```python
from build123d import *

# Parameters (mm, degrees)
F1_DEPTH = 6.35
F2_R     = 15.875
F2_R_2   = 8.7674107973
F3_DEPTH = 6.35


# Not quite as in the source:
# - a feature names something its author has since deleted; it is built from what else it names


with BuildPart() as f1:
    # F0 (on Front) → F1 (new body)
    with BuildSketch(Plane.XZ):
        Polygon((-15.875, 25.1552741975), (-50.8, 8.7795666171), (-50.8, -35.6704333829), (0, -35.6704333829), (0, 25.1552741975), align=None)
        Polygon((0, 25.1552741975), (0, -35.6704333829), (50.8, -35.6704333829), (50.8, 8.7795666171), (15.875, 25.1552741975), align=None)
    extrude(amount=F1_DEPTH)

    # F2 (on face) → F3 (cut)
    with BuildSketch(Plane.XZ.offset(6.35)):
        with Locations((0, -3.9204333829)):
            Circle(F2_R)
        with Locations((31.75, -16.6204333829)):
            Circle(F2_R_2)
        with Locations((-31.75, -16.6204333829)):
            Circle(F2_R_2)
    extrude(amount=-F3_DEPTH, mode=Mode.SUBTRACT)


solid = f1.part
```
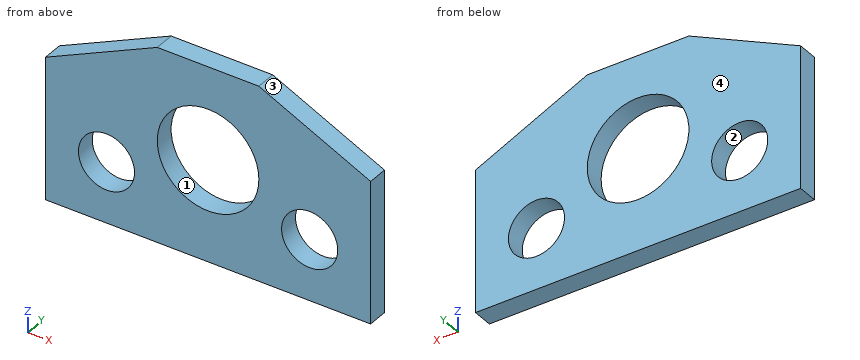
Part model, mm, in its own coordinate system. Face numbers are marked on the shaded views. Give positions to 0.01 mm unless a question says otherwise; leave off trailing zeros. Write each loop counter-clockwise with the first axis right and the second up, starting at its lowest first coordinate (ties: lowest second). Pieces come first, ordered by that corner, then holes. Notation, with made-up numbers: (60, 28.25) -> (77, 28.25) arc R23 cw to (77, 56.25) -> close; hole circle Ø11 at (30.5, 36). An arc over 180 degrees is marked (long way). Put each result on its own line as item: value. Start each with the question number.
Item 1: Pin check, flat tip, straight feed: pin 1 Ø3 at (x, y) = (20.5, -2.5) entering from +Z. Stop position of the tip, or through.
Item 2: Cut at C-C (z = -2.5). List the corners of the cut face in (x, y), then the cut area to 3 significant figures.
Item 3: Cut at D-D (z = 16). List the corners of the cut face in (x, y).
Item 4: Cut at B-B (y = -4.75). List the corners of the cut face in (x, z) (3 decimals), then the cut area to 3 significant figures.
Item 5: Wall check: L1, parallel to X at y = -5.5, z = -16; L2, parallel to X at y = -0.75, z = -4.5; L3, parallel to Z at x = 0.5, y = -0.5. Give the ranges that are in metal, low to high. Write a range as [from, to].
Item 6: Cut at A-A (x = 0). List the corners of the cut face in (y, z).
Item 7: Pull direction Z, two halves, no side cores. Call the marked faces 1, 2, 3 and 4: pulls with the +Z half, pulls with the -Z half, needs draft (parallel to the pull), parting line crosses it, or undercut.
Answer list:
1. pin 1: stops at z = 23.69
2. outline: (-50.8, -6.35) -> (-15.81, -6.35) -> (-15.81, 0) -> (-50.8, 0) -> close; (15.81, -6.35) -> (50.8, -6.35) -> (50.8, 0) -> (15.81, 0) -> close
2. area: 444 mm2
3. outline: (-35.4, -6.35) -> (35.4, -6.35) -> (35.4, 0) -> (-35.4, 0) -> close
4. outline: (-50.8, -35.67) -> (50.8, -35.67) -> (50.8, 8.78) -> (15.875, 25.155) -> (-15.875, 25.155) -> (-50.8, 8.78) -> close; hole circle Ø17.535 at (-31.75, -16.62); hole circle Ø31.75 at (0, -3.92); hole circle Ø17.535 at (31.75, -16.62)
4. area: 4,330 mm2
5. L1: x = [-50.8, -40.5], [-23, -10.3], [10.3, 23], [40.5, 50.8]
5. L2: x = [-50.8, -15.86], [15.86, 50.8]
5. L3: z = [-35.67, -19.79], [11.95, 25.16]
6. outline: (-6.35, -35.67) -> (0, -35.67) -> (0, -19.8) -> (-6.35, -19.8) -> close; (-6.35, 11.95) -> (0, 11.95) -> (0, 25.16) -> (-6.35, 25.16) -> close
7. face 1: undercut
7. face 2: undercut
7. face 3: pulls with the +Z half
7. face 4: needs draft
